```python
from build123d import *

# Parameters (mm, degrees)
F0_W      = 215
F0_H      = 30
F0_W_2    = 300
F3_DEPTH  = 15
F5_DEPTH  = 15
F8_DEPTH  = 12.7
F11_DEPTH = 12.7
F13_D     = 12.5
F13_DEPTH = 25.4
F13_TIP   = 3.7553788689
F14_R     = 75
F15_DEPTH = 200


with BuildPart() as f1:
    # F0 (on Right) → F1 (revolve)
    with BuildSketch(Plane.YZ):
        with Locations((107.5, 0)):
            Rectangle(F0_W, F0_H)
    revolve(axis=Axis((0, 0, 0), (0, 0, 1)))



with BuildPart() as f2:
    # F0 (on Right) → F2 (revolve)
    with BuildSketch(Plane.YZ):
        with Locations((150, 170)):
            Rectangle(F0_W_2, F0_H)
    revolve(axis=Axis((0, 0, 170), (0, 0, 1)))


with BuildPart() as f1_1:
    add(f1.part)

    add(f2.part)  # F3 merges F2
    # F0 (on Right) → F3 (join, symmetric)
    with BuildSketch(Plane.YZ):
        Polygon((-215, 15), (0, 15), (0, 155), (-300, 155), align=None)
        Polygon((0, 15), (215, 15), (300, 155), (0, 155), align=None)
    extrude(amount=F3_DEPTH, both=True)

    # F4 (on Front) → F5 (join, symmetric)
    with BuildSketch(Plane.XZ):
        Polygon((0, 15), (215, 15), (300, 155), (0, 155), align=None)
        Polygon((-215, 15), (0, 15), (0, 155), (-300, 155), align=None)
    extrude(amount=F5_DEPTH, both=True)

    # F7 (on line) → F8 (join, symmetric)
    with BuildSketch(Plane(origin=(0, 0, 0), x_dir=(-0.7071067812, 0.7071067812, 0), z_dir=(0.7071067812, 0.7071067812, 0))):
        Polygon((-215, 15), (215, 15), (300, 155), (-300, 155), align=None)
    extrude(amount=F8_DEPTH, both=True)

    # F10 (on line) → F11 (join, symmetric)
    with BuildSketch(Plane(origin=(0, 0, 0), x_dir=(0.7071067812, 0.7071067812, 0), z_dir=(0.7071067812, -0.7071067812, 0))):
        Polygon((-215, 15), (215, 15), (300, 155), (-300, 155), align=None)
    extrude(amount=F11_DEPTH, both=True)

    # F13
    with Locations(Plane(origin=(0, 0, -15), x_dir=(1, 0, 0), z_dir=(0, 0, -1))):
        with Locations((-187.7323210063, 77.7612734566), (-77.7612734566, 187.7323210063), (77.7612734566, 187.7323210063), (187.7323210063, 77.7612734566), (187.7323210063, -77.7612734566), (77.7612734566, -187.7323210063), (-77.7612734566, -187.7323210063), (-187.7323210063, -77.7612734566), (-93.8661605031, -38.8806367283), (-38.8806367283, -93.8661605031), (38.8806367283, -93.8661605031), (93.8661605031, -38.8806367283), (93.8661605031, 38.8806367283), (38.8806367283, 93.8661605031), (-38.8806367283, 93.8661605031), (-93.8661605031, 38.8806367283)):
            Hole(F13_D / 2, depth=F13_DEPTH)
            with Locations((0, 0, -(F13_DEPTH + F13_TIP / 2))):  # 118° drill point
                Cone(0, F13_D / 2, F13_TIP, mode=Mode.SUBTRACT)

    # F14 (on face) → F15 (join)
    with BuildSketch(Plane(origin=(0, 0, -15), x_dir=(1, 0, 0), z_dir=(0, 0, -1))):
        Circle(F14_R)
    extrude(amount=-F15_DEPTH)


solid = f1_1.part
```
Verification items for the finished model (mm, model axes). A direction names the side the tool comes from. Coordinates: 2 decimals unless noted, no trailing zeros. Order: outer loops, then holes, each group sorted by start corner. A loop starts at its lowest first (then second) coordinate and runs counter-clockwise, first axis right, second up. Notation, with made-up numbers: (87.5, 82.25) -> (135.5, 82.25) arc R30 ccw to (135.5, 108.25) -> close; hole circle Ø2 at (84.25, -1). An arc over 180 degrees is marked (long way). Answer as CSV lines item,"result". Start each with the question number.
1) Release check for a two-part mould opening along Z. For faces 6 (the face through (0.21, -258.095, 85.98)), 7 (the face through (87, 182, 155)) record: released by +Z, released by -Z, zero draft, split by the parting line, or undercut.
2) Cross-section at D-D, the plane x = -259.5. Record the boundary of the cut face in (y, z).
3) Set-up check for faces 1 (the face through (-3, -3, -15)), 2 (the face through (130.82, -170.62, 0.21)), 3 (the face through (-29.58, -68.92, 84.02)), 4 (the face through (137, -64, 15)), 5 (the face through (104.34, 122.3, 85.98)): record each of +Z, -Z, +X, -X, +Y, -Y from which the full face is reachable in a straight line by a thin tool's end or side.
4) Material ranges on L1, parallel to X at y = -80, z = 66; L2, parallel to Z at x = 128.5, y = -41; L3, parallel to Y at x = -164.5, z = 124.5, recorded low to high. Write a range as [from, to].
5) Cross-section at A-A, the plane x = -108. Record the boundary of the cut face in (y, z), then the cut area to 3 significant figures.
6) Cross-section at B-B, the plane y = -245. Record the boundary of the cut face in (x, z), then the cut area to 3 significant figures.
7) Gauge pin test, flat ends, axial feed: pin 1 Ø1.5 at (x, z) = (-121, 87) entering from +Y; pin 2 Ø1 at (x, z) = (-135.5, 10) entering from -Y; pin 3 Ø16 at (x, y) = (93.87, 38.88) entering from -Z; pin 4 Ø12 at (y, z) = (182.5, 160) entering from +X. Record the tip position at first contact, or that the pin passes through.
Conclusion:
1,face 6,"released by -Z"
1,face 7,"undercut"
2,outline,"(-150.53, 155) -> (-15, 155) -> (-15, 88.29) -> (15, 88.29) -> (15, 155) -> (150.53, 155) -> (150.53, 185) -> (-150.53, 185) -> close"
3,face 1,"-Z, +X, -X, +Y, -Y"
3,face 2,"-Z"
3,face 3,"-Y"
3,face 4,"+X"
3,face 5,"+Y"
4,L1,"x = [-97.96, -62.04], [-15, 15], [62.04, 97.96]"
4,L2,"z = [-15, 15], [155, 185]"
4,L3,"y = [-182.46, -146.54], [-15, 15], [146.54, 182.46]"
5,outline,"(-279.89, 155) -> (-125.96, 155) -> (-125.96, 15) -> (-185.91, 15) -> (-185.91, -15) -> (185.91, -15) -> (185.91, 15) -> (125.96, 15) -> (125.96, 155) -> (279.89, 155) -> (279.89, 185) -> (-279.89, 185) -> close; hole (-90.04, 15) -> (-15, 15) -> (-15, 155) -> (-90.04, 155) -> close; hole (15, 15) -> (90.04, 15) -> (90.04, 155) -> (15, 155) -> close"
5,area,"42,200 mm²"
6,outline,"(-173.13, 155) -> (-15, 155) -> (-15, 64.41) -> (15, 64.41) -> (15, 155) -> (173.13, 155) -> (173.13, 185) -> (-173.13, 185) -> close"
6,area,"13,100 mm²"
7,pin 1,"stops at y = 139.71"
7,pin 2,"stops at y = -167.33"
7,pin 3,"stops at z = -15"
7,pin 4,"stops at x = 242.59"
